from build123d import *

# Parameters (mm, degrees)
SKETCH1_R                = 32.5
SKETCH1_R_2              = 25
SKETCH1_R_3              = 1
RING_BODY_DEPTH          = 10
SKETCH2_R                = 6
NUB_CUT_DEPTH            = 6.5
NUB_CUT_FILLETS_3MM_R    = 3
WEIGHT_REDUCTION_DEPTH   = 7
WEIGHT_REDUCTION_2_DEPTH = 0.5


# Read off the part's stored shape, not the designer's step: Weight reduction
with BuildPart() as part:
    # Sketch1 → Ring body (new body)
    with BuildSketch(Plane.XY):
        Circle(SKETCH1_R)
        Circle(SKETCH1_R_2, mode=Mode.SUBTRACT)
        with Locations((0, 27.5)):
            Circle(SKETCH1_R_3, mode=Mode.SUBTRACT)
        with Locations((23.5226917, 14.245454545)):
            Circle(SKETCH1_R_3, mode=Mode.SUBTRACT)
        with Locations((-27.5, 0)):
            Circle(SKETCH1_R_3, mode=Mode.SUBTRACT)
        with Locations((-11.677272727, -24.897616385)):
            Circle(SKETCH1_R_3, mode=Mode.SUBTRACT)
    extrude(amount=RING_BODY_DEPTH)

    # Sketch2 → Nub cut (cut)
    with BuildSketch(Plane.XY.offset(10)):
        with Locations((25, 0)):
            Circle(SKETCH2_R)
    extrude(amount=-NUB_CUT_DEPTH, mode=Mode.SUBTRACT)

    # Nub cut fillets 3mm
    nub_cut_fillets_3mm_edges = [part.edges().sort_by_distance(p)[0] for p in [
        (24.28, 5.95664335, 6.75),
        (24.28, -5.95664335, 6.75),
    ]]
    fillet(nub_cut_fillets_3mm_edges, radius=NUB_CUT_FILLETS_3MM_R)

    # Weight reduction outline → Weight reduction (cut)
    with BuildSketch(Plane.XY):
        with BuildLine():
            ThreePointArc((32.005, -5.650661466), (29.573928418, -7.751075978), (26.56, -8.86376895))
            ThreePointArc((26.56, -8.86376895), (12.846329016, -24.879144495), (-8.151686125, -26.787124021))
            ThreePointArc((-8.151686125, -26.787124021), (-13.375785124, -28.519087859), (-15.384291336, -23.394947747))
            ThreePointArc((-15.384291336, -23.394947747), (-23.631635891, -15.018181818), (-27.713636364, -3.994290864))
            ThreePointArc((-27.713636364, -3.994290864), (-31.5, 0), (-27.713636364, 3.994290864))
            ThreePointArc((-27.713636364, 3.994290864), (-19.798989873, 19.798989873), (-3.994290864, 27.713636364))
            ThreePointArc((-3.994290864, 27.713636364), (0, 31.5), (3.994290864, 27.713636364))
            ThreePointArc((3.994290864, 27.713636364), (13.745454545, 24.393902503), (21.636321277, 17.772720715))
            ThreePointArc((21.636321277, 17.772720715), (26.944174129, 16.317520661), (25.774538654, 10.939522711))
            ThreePointArc((25.774538654, 10.939522711), (26.187843982, 9.909431242), (26.56, 8.86376895))
            ThreePointArc((26.56, 8.86376895), (29.573928418, 7.751075978), (32.005, 5.650661466))
            ThreePointArc((32.005, 5.650661466), (-32.5, 0), (32.005, -5.650661466))
        make_face()
    extrude(amount=WEIGHT_REDUCTION_DEPTH, mode=Mode.SUBTRACT)

    # Weight reduction 2 outline → Weight reduction 2 (cut)
    with BuildSketch(Plane.XY):
        with BuildLine():
            ThreePointArc((26.56, 8.86376895), (28, 0), (26.56, -8.86376895))
            ThreePointArc((26.56, -8.86376895), (29.573928418, -7.751075978), (32.005, -5.650661466))
            ThreePointArc((32.005, -5.650661466), (32.5, 0), (32.005, 5.650661466))
            ThreePointArc((32.005, 5.650661466), (29.573928418, 7.751075978), (26.56, 8.86376895))
        make_face()
    extrude(amount=WEIGHT_REDUCTION_2_DEPTH, mode=Mode.SUBTRACT)


solid = part.part
Here's how the part is built. I have some questions about the finished solid (model axes, mm). A direction names the side the tool comes from. Round coordinates to 2 decimals unless told otherwise and drop trailing zeros. Order: outer loops, then holes, each group sorted by start corner. A loop starts at its lowest first (then second) coordinate and runs counter-clockwise, first axis right, second up. Notation, with made-up numbers: M -13.75,19.5 L 12.25,19.5 A14 cw 12.25,40.5 Z; hole C -7.5,25.5 d1. An arc over 180 degrees is marked long. Return JSON: item names as keys, results as strings. Group by question number.
1. If we section it at C-C on x = -21: List the corners of the cut face in (y, z) for me, then the cut area to 3 significant figures.
2. If we section it at B-B on y = 12.5: List the corners of the cut face in (x, z) for me, then the cut area to 3 significant figures.
3. On a 3-axis mill with a long thin cutter (end or side, diameter ignored), from which of +Z, -Z, +X, -X, +Y, -Y can I reach the whole of each face in a straight line? I mean faces 1 (the face through (-31.5, -0.1, 3.5)), 2 (the face through (27, 0, 3.5)), 3 (the face through (-13, 22, 0)), 4 (the face through (29.61, -7.73, 3.7)), 5 (the face through (26.9, 16.39, 3.45)). Say none if no direction works.
4. If we section it at D-D on z = 7.75: State how many separate pieces and enclosed holes the cut face has, then the cut area to 3 significant figures.
5. If we section it at A-A on x = 0: List the corners of the cut face in (y, z) for me.
6. I'm going to push flat-ended pins straight in: pin 1 Ø3 at (x, y) = (-22.5, -24.5) entering from +Z; pin 2 Ø3.5 at (x, y) = (26.5, 1) entering from +Z; pin 3 Ø3 at (y, z) = (-12, 7) entering from +X; pin 4 Ø2 at (x, z) = (-23.5, 4.5) entering from +Y. Where does each tip first touch, or does it pass through?
7. Please list where these lines run through material, in increasing order: probe 1 along X at (y, z) = (15, 9); probe 2 along Z at (x, y) = (-26, -15.5); probe 3 along X at (y, z) = (0.5, 1.5) (3 decimals).
8. If we mould it in two halves opening along Y, with no side actions, what happens to faces 6 (the face through (-28.5, 0, 4.9)), 7 (the face through (23.31, 13.27, 4.93)), 8 (the face through (-0.1, 31.5, 3.5)), 9 (the face through (32.332, 3.299, 8.043))? For each: pulls with the +Y half, pulls with the -Y half, needs draft (parallel to the pull), parting line crosses it, or undercut.
Reply:
{
 "1": {"outline": "M -24.8,7 L -18.52,7 L -18.52,0 L -13.56,0 L -13.56,10 L -24.8,10 Z; M 13.56,0 L 18.52,0 L 18.52,7 L 24.8,7 L 24.8,10 L 13.56,10 Z", "area": "137 mm^2"},
 "2": {"outline": "M -30,7 L -25.05,7 L -25.05,0 L -21.65,0 L -21.65,10 L -30,10 Z; M 21.65,0 L 27.12,0 L 27.12,7 L 30,7 L 30,10 L 21.65,10 Z", "area": "112 mm^2"},
 "3": {"face 1": "-Z, -X", "face 2": "+Z", "face 3": "-Z, +X, -X, +Y, -Y", "face 4": "-Z, +X, -Y", "face 5": "-Z"},
 "4": {"separate pieces": "1", "enclosed holes": "5", "area": "1,280 mm^2"},
 "5": {"outline": "M -32.5,7 L -28,7 L -28,0 L -25,0 L -25,10 L -32.5,10 Z; M 25,0 L 26.5,0 L 26.5,10 L 25,10 Z; M 28.5,0 L 31.5,0 L 31.5,7 L 32.5,7 L 32.5,10 L 28.5,10 Z"},
 "6": {"pin 1": "z = 10", "pin 2": "z = 3.5", "pin 3": "x = 30.76", "pin 4": "y = 16.67"},
 "7": {"probe 1": "-28.83 to -20, 20 to 22.87, 24.18 to 28.83", "probe 2": "7 to 10", "probe 3": "-31.469 to -28.366, -26.634 to -24.995, 24.995 to 32.496"},
 "8": {"face 6": "undercut", "face 7": "undercut", "face 8": "pulls with the +Y half", "face 9": "parting line crosses it"}
}
